Design review of the part built by this model. Coordinates are the model's own, in mm. A direction names the side the tool comes from. Round coordinates to 2 decimals unless told otherwise and drop trailing zeros. Write each loop counter-clockwise with the first axis right and the second up, starting at its lowest first coordinate (ties: lowest second). Pieces come first, ordered by that corner, then holes. Notation, with made-up numbers: (45, 5) - (86, 5) arc R9 cw to (86, 18) - close; hole circle Ø5 at (55, -0.75). An arc over 180 degrees is marked (long way). Use one line per item in the form item = value.
```python
from build123d import *

# Parameters (mm, degrees)
SKETCH2_R             = 52.5
SKETCH2_R_2           = 47.5
BOSS_EXTRUDE1_DEPTH   = 20
SKETCH2_R_3           = 77.5
SKETCH2_R_4           = 72.5
BOSS_EXTRUDE1_2_DEPTH = 20
SKETCH3_R             = 77.5
BOSS_EXTRUDE2_DEPTH   = 5


with BuildPart() as part:
    # Sketch2 → Boss-Extrude1 (new body)
    with BuildSketch(Plane(origin=(0, 0, 0), x_dir=(1, 0, 0), z_dir=(0, 1, 0))):
        Circle(SKETCH2_R)
        Circle(SKETCH2_R_2, mode=Mode.SUBTRACT)
    extrude(amount=BOSS_EXTRUDE1_DEPTH)



with BuildPart() as body_2:
    # Sketch2 → Boss-Extrude1 2 (new body)
    with BuildSketch(Plane(origin=(0, 0, 0), x_dir=(1, 0, 0), z_dir=(0, 1, 0))):
        Circle(SKETCH2_R_3)
        Circle(SKETCH2_R_4, mode=Mode.SUBTRACT)
    extrude(amount=BOSS_EXTRUDE1_2_DEPTH)


with BuildPart() as part_1:
    add(part.part)

    add(body_2.part)  # Boss-Extrude2 merges body 2
    # Sketch3 → Boss-Extrude2 (add)
    with BuildSketch(Plane(origin=(0, 20, 0), x_dir=(1, 0, 0), z_dir=(0, 1, 0))):
        Circle(SKETCH3_R)
    extrude(amount=BOSS_EXTRUDE2_DEPTH)


solid = part_1.part
```
Q1. Draft analysis for pull direction Z (two halves, no side actions). For faces 3 (the cylindrical face through (-16.8, 12.325, 75.657)), 4 (the flat face through (-1, 25, -1)), 5 (the flat face through (48, 20, -22)), 6 (the flat face through (-1, 20, -1)), state which applies: released by +Z, released by -Z, zero draft, split by the parting line, or undercut.
Calculated:
face_3 = split by the parting line
face_4 = zero draft
face_5 = undercut
face_6 = undercut
Q2. We need section A-A on y = 12. Write out the cut boundary in (x, z), then the cut area to 3 significant figures.
Calculated:
outline = circle Ø155 at (0, 0); circle Ø105 at (0, 0); hole circle Ø145 at (0, 0); hole circle Ø95 at (0, 0)
area = 3,930 mm2
Q3. We need section B-B on x = 0. Write out the cut boundary in (y, z).
Calculated:
outline = (0, -77.5) - (25, -77.5) - (25, 77.5) - (0, 77.5) - (0, 72.5) - (20, 72.5) - (20, 52.5) - (0, 52.5) - (0, 47.5) - (20, 47.5) - (20, -47.5) - (0, -47.5) - (0, -52.5) - (20, -52.5) - (20, -72.5) - (0, -72.5) - close
Q4. For P1, Ø6, axis at x = 8, y = 14.5, coming from the +Z side; P2, Ø1.5, axis at x = 23, y = 12.5, coming from the +Z side; P3, Ø1, axis at x = -44, y = 9.5, coming from the -Z side, all flat-tipped, find the tip position at first contact; note any pin that passes through.
Calculated:
P1 = 77.34
P2 = 74.24
P3 = -64.14
Q5. We need section D-D on z = -66. Write out the cut boundary in (x, y).
Calculated:
outline = (-40.62, 0) - (-30, 0) - (-30, 20) - (30, 20) - (30, 0) - (40.62, 0) - (40.62, 25) - (-40.62, 25) - close
Q6. Machinability: for faces 1 (the cylindrical face through (-10.3, 9.86, 46.37)), 2 (the flat face through (-11.9, 0, 46.4)), which of the approach directions +Z, -Z, +X, -X, +Y, -Y give a long, thin tool a straight path to every point of the face, cutting with its end or side? Answer none if there is none.
Calculated:
face_1 = -Y
face_2 = +Z, -Z, +X, -X, -Y
Q7. To check wall thickness, follow line 1 along Z through (x, y) = (0, 15.75); line 2 along Z through (x, y) = (11.5, 13) (3 decimals). State the ranges of each line that lie inside material, in increasing order. Write a range as from..to.
Calculated:
line_1 = -77.5..-72.5, -52.5..-47.5, 47.5..52.5, 72.5..77.5
line_2 = -76.642..-71.582, -51.225..-46.087, 46.087..51.225, 71.582..76.642
Q8. We need section C-C on z = 0. Write out the cut boundary in (x, y).
Calculated:
outline = (-77.5, 0) - (-72.5, 0) - (-72.5, 20) - (-52.5, 20) - (-52.5, 0) - (-47.5, 0) - (-47.5, 20) - (47.5, 20) - (47.5, 0) - (52.5, 0) - (52.5, 20) - (72.5, 20) - (72.5, 0) - (77.5, 0) - (77.5, 25) - (-77.5, 25) - close
